Part model, mm, in its own coordinate system. Face numbers are marked on the shaded views. A direction names the side the tool comes from. Round coordinates to 2 decimals unless told otherwise and drop trailing zeros. Write each loop counter-clockwise with the first axis right and the second up, starting at its lowest first coordinate (ties: lowest second). Pieces come first, ordered by that corner, then holes.
1) Saw through at A-A on z = 0. Write the cut outline in (x, y).
2) Saw through at B-B on x = 22.5. Write the cut outline in (y, z), and give its area (3 significant figures).
3) Pull direction X, two halves, no side cores. Call the marked faces 3, 4 and 5: +X half, -X half, draft (parallel to the pull), parting line (faces both ways), or undercut.
4) Saw through at C-C on y = 1. Write the cut outline in (x, z).
5) Saw through at D-D on z = -7.5. Write the cut outline in (x, y), and give its area (3 significant figures).
6) Drill centre lines: L1, parallel to Z at x = -15, y = 0; L2, parallel to Z at x = -15, y = -3.1; L3, parallel to X at y = -4, z = 2.25. Where is each one in solid material? Low to high.
7) Which spindle directions (+Z, -Z, +X, -X, +Y, -Y) get a long thin tool onto all of the face, cutting with end or side? Do the marked faces 1 and 2. Say none if no direction does.
8) Flat gauge pin, fed straight in: pin 1 (5.5 mm diameter, centred on x = 21, z = 2, fed in from +Y). Where does the tip first touch, or does it go through?
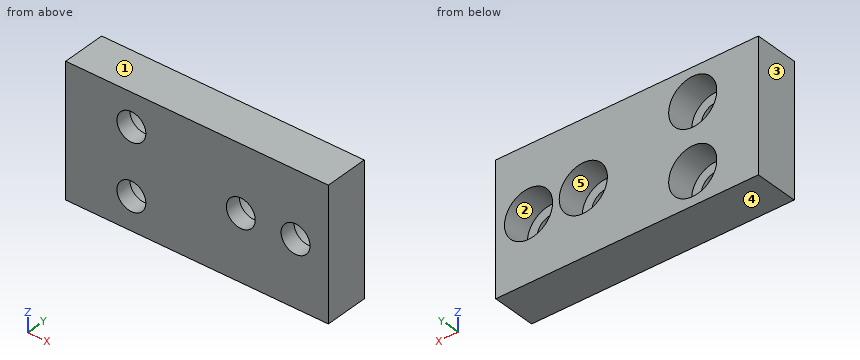
```python
from build123d import *

# Parameters (mm, degrees)
SKETCH1_W                                           = 60
SKETCH1_H                                           = 30
BOSS_EXTRUDE1_DEPTH                                 = 5
CBORE_FOR_M6_HEX_SOCKET_HEAD_CAP_SCREW1_D           = 6.6
CBORE_FOR_M6_HEX_SOCKET_HEAD_CAP_SCREW1_CBORE_D     = 11
CBORE_FOR_M6_HEX_SOCKET_HEAD_CAP_SCREW1_CBORE_DEPTH = 6.4
CBORE_FOR_M6_HEX_SOCKET_HEAD_CAP_SCREW2_D           = 6.6
CBORE_FOR_M6_HEX_SOCKET_HEAD_CAP_SCREW2_CBORE_D     = 11
CBORE_FOR_M6_HEX_SOCKET_HEAD_CAP_SCREW2_CBORE_DEPTH = 6.4


with BuildPart() as part:
    # Sketch1 → Boss-Extrude1 (new, symmetric)
    with BuildSketch(Plane(origin=(0, 0, 0), x_dir=(1, 0, 0), z_dir=(0, 1, 0))):
        Rectangle(SKETCH1_W, SKETCH1_H)
    extrude(amount=BOSS_EXTRUDE1_DEPTH, both=True)

    # CBORE for M6 Hex Socket Head Cap Screw1 (through all)
    with Locations(Plane(origin=(0, 5, 0), x_dir=(1, 0, 0), z_dir=(0, 1, 0))):
        with Locations((-15, 7.5), (-15, -7.5)):
            CounterBoreHole(CBORE_FOR_M6_HEX_SOCKET_HEAD_CAP_SCREW1_D / 2, CBORE_FOR_M6_HEX_SOCKET_HEAD_CAP_SCREW1_CBORE_D / 2, CBORE_FOR_M6_HEX_SOCKET_HEAD_CAP_SCREW1_CBORE_DEPTH)

    # CBORE for M6 Hex Socket Head Cap Screw2 (through all)
    with Locations(Plane(origin=(0, 5, 0), x_dir=(1, 0, 0), z_dir=(0, 1, 0))):
        with Locations((10, 0), (22.5, 0)):
            CounterBoreHole(CBORE_FOR_M6_HEX_SOCKET_HEAD_CAP_SCREW2_D / 2, CBORE_FOR_M6_HEX_SOCKET_HEAD_CAP_SCREW2_CBORE_D / 2, CBORE_FOR_M6_HEX_SOCKET_HEAD_CAP_SCREW2_CBORE_DEPTH)


solid = part.part
```
Completed:
1. outline: (-30, -5) - (6.7, -5) - (6.7, -1.4) - (4.5, -1.4) - (4.5, 5) - (-30, 5) - close; (13.3, -5) - (19.2, -5) - (19.2, -1.4) - (17, -1.4) - (17, 5) - (15.5, 5) - (15.5, -1.4) - (13.3, -1.4) - close; (25.8, -5) - (30, -5) - (30, 5) - (28, 5) - (28, -1.4) - (25.8, -1.4) - close
2. outline: (-5, -15) - (5, -15) - (5, -5.5) - (-1.4, -5.5) - (-1.4, -3.3) - (-5, -3.3) - close; (-5, 3.3) - (-1.4, 3.3) - (-1.4, 5.5) - (5, 5.5) - (5, 15) - (-5, 15) - close
2. area: 206 mm2
3. face 3: -X half
3. face 4: draft
3. face 5: undercut
4. outline: (-30, -15) - (30, -15) - (30, 15) - (-30, 15) - close; hole circle Ø11 at (-15, -7.5); hole circle Ø11 at (-15, 7.5); hole circle Ø11 at (10, 0); hole circle Ø11 at (22.5, 0)
5. outline: (-30, -5) - (-18.3, -5) - (-18.3, -1.4) - (-20.5, -1.4) - (-20.5, 5) - (-30, 5) - close; (-11.7, -5) - (30, -5) - (30, 5) - (-9.5, 5) - (-9.5, -1.4) - (-11.7, -1.4) - close
5. area: 506 mm2
6. L1: z = -15 to -13, -2 to 2, 13 to 15
6. L2: z = -15 to -10.8, -4.2 to 4.2, 10.8 to 15
6. L3: x = -30 to 7.59, 12.41 to 20.09, 24.91 to 30
7. face 1: +Z, +X, -X, +Y, -Y
7. face 2: +Y
8. pin 1: stops at y = -1.4
